```python
from build123d import *

# Parameters (mm, degrees)
F1_DEPTH = 7.5
F3_DEPTH = 7.5
F4_R     = 15
F5_R     = 25
F7_DEPTH = 2


with BuildPart() as f1:
    # F0 (on Front) → F1 (new body, symmetric)
    with BuildSketch(Plane.XZ):
        with BuildLine():
            Line((15.571662, 31.4), (-31.4, 31.4))
            Line((-31.4, 31.4), (-31.4, -31.016811))
            ThreePointArc((-31.4, -31.016811), (-31.146187, -31.209444), (-30.890811, -31.4))
            Line((-30.890811, -31.4), (15.571662, -31.4))
            ThreePointArc((15.571662, -31.4), (31.4, 0), (15.571662, 31.4))
        make_face()
        with BuildLine():
            Line((-21.4, -21.4), (-21.4, 21.4))
            Line((-21.4, 21.4), (12, 21.4))
            ThreePointArc((12, 21.4), (21.4, 0), (12, -21.4))
            Line((12, -21.4), (-21.4, -21.4))
        make_face(mode=Mode.SUBTRACT)
        with BuildLine():
            ThreePointArc((-30.890811, -31.4), (-31.146187, -31.209444), (-31.4, -31.016811))
            Line((-31.4, -31.016811), (-31.4, -31.4))
            Line((-31.4, -31.4), (-30.890811, -31.4))
        make_face()
    extrude(amount=F1_DEPTH, both=True)

    # F2 (on Front) → F3 (join, symmetric)
    with BuildSketch(Plane.XZ):
        with BuildLine():
            ThreePointArc((-71, 31.4), (-93.271008, 0), (-71, -31.4))
            Line((-71, -31.4), (-31.4, -31.4))
            Line((-31.4, -31.4), (-31.4, 6))
            Line((-31.4, 6), (-60, 6))
            Line((-60, 6), (-60, -4))
            Line((-60, -4), (-41.4, -4))
            Line((-41.4, -4), (-41.4, -21.4))
            Line((-41.4, -21.4), (-71, -21.4))
            ThreePointArc((-71, -21.4), (-83.271008, 0), (-71, 21.4))
            Line((-71, 21.4), (-31.4, 21.4))
            Line((-31.4, 21.4), (-31.4, 31.4))
            Line((-31.4, 31.4), (-71, 31.4))
        make_face()
    extrude(amount=F3_DEPTH, both=True)

    # F4
    f4_edges = [f1.edges().sort_by_distance(p)[0] for p in [
        (-71, 0, 21.4),
        (-71, 0, -21.4),
        (12, 0, -21.4),
        (12, 0, 21.4),
    ]]
    fillet(f4_edges, radius=F4_R)

    # F5
    f5_edges = [f1.edges().sort_by_distance(p)[0] for p in [
        (-71, 0, 31.4),
        (-71, 0, -31.4),
        (15.571662, 0, -31.4),
        (15.571662, 0, 31.4),
    ]]
    fillet(f5_edges, radius=F5_R)

    # F6 (on Front) → F7 (cut, symmetric)
    with BuildSketch(Plane.XZ):
        with BuildLine():
            Line((-22.9, 35.188502), (-22.9, 0))
            ThreePointArc((-22.9, 0), (0, -22.9), (22.9, 0))
            Line((22.9, 0), (22.9, 35.188502))
            Line((22.9, 35.188502), (-22.9, 35.188502))
        make_face()
    extrude(amount=F7_DEPTH, both=True, mode=Mode.SUBTRACT)


solid = f1.part
```
Model file for the job. Use its own axes, mm. A direction names the side the tool comes from. Coordinates: 2 decimals unless noted, no trailing zeros. Order: outer loops, then holes, each group sorted by start corner. A loop starts at its lowest first (then second) coordinate and runs counter-clockwise, first axis right, second up. Notation, with made-up numbers: M 52.25,75 L 74.25,75 A30 cw 74.25,109 Z; hole C 30.25,-35 d9. An arc over 180 degrees is marked long. Answer as CSV lines item,"result".
(1) Flat gauge pins, fed straight in: pin 1 (1 mm diameter, centred on x = -80.5, z = -5.5, fed in from +Y); pin 2 (5 mm diameter, centred on y = 0.5, z = -11.5, fed in from +X); pin 3 (2 mm diameter, centred on y = -0.5, z = 11, fed in from -X); pin 4 (4.5 mm diameter, centred on y = -3, z = -15, fed in from -X). Where does each tip first touch, or does it go through?
Geometry says:
pin 1,"passes through"
pin 2,"stops at x = 30.35"
pin 3,"stops at x = -91.73"
pin 4,"stops at x = -90.73"
(2) Band-saw the part on D-D, the plane x = -13.5. List the corners of the cut face in (y, z), then the cut area to 3 significant figures.
Geometry says:
outline,"M -7.5,-31.4 L 7.5,-31.4 L 7.5,-21.4 L -7.5,-21.4 Z; M -7.5,21.4 L -2,21.4 L -2,31.4 L -7.5,31.4 Z; M 2,21.4 L 7.5,21.4 L 7.5,31.4 L 2,31.4 Z"
area,"260 mm2"
(3) Band-saw the part on C-C, the plane z = -6.5. List the corners of the cut face in (x, y).
Geometry says:
outline,"M -92.63,-7.5 L -82.4,-7.5 L -82.4,7.5 L -92.63,7.5 Z; M -41.4,-7.5 L -21.4,-7.5 L -21.4,-2 L -21.96,-2 L -21.96,2 L -21.4,2 L -21.4,7.5 L -41.4,7.5 Z; M 20.66,-7.5 L 30.86,-7.5 L 30.86,7.5 L 20.66,7.5 L 20.66,2 L 21.96,2 L 21.96,-2 L 20.66,-2 Z"
(4) 3-axis set-ups, long thin cutter, end or side, ignore diameter. For faces 5 (the flat face through (0, 2, 22)), 6 (the flat face through (-30, 0, 31.4)), 7 (the cylindrical face through (21.4, -4.8, 0.2)): which of +Z, -Z, +X, -X, +Y, -Y reach the whole face in a straight line?
Geometry says:
face 5,"+Z"
face 6,"+Z, +X, -X, +Y, -Y"
face 7,"+Y, -Y"
(5) Band-saw the part on A-A, the plane y = -0.25. List the corners of the cut face in (x, z), then the cut area to 3 significant figures.
Geometry says:
outline,"M -81.08,-25.74 A25 ccw -65.24,-31.4 L 4.86,-31.4 A25 ccw 27.12,-17.78 A39.06 ccw 27.12,17.78 A25 ccw 22.9,23.71 L 22.9,0 A22.9 cw 16.39,-15.99 A15 cw 11,-20.09 A22.9 cw -8.15,-21.4 L -21.4,-21.4 L -21.4,-8.15 A22.9 cw -22.9,0 L -22.9,31.4 L -65.24,31.4 A25 ccw -81.08,25.74 A33.27 ccw Z; hole M -77.25,-16.2 A15 ccw -65.89,-21.4 L -41.4,-21.4 L -41.4,-4 L -60,-4 L -60,6 L -31.4,6 L -31.4,21.4 L -65.89,21.4 A15 ccw -77.25,16.2 A24.8 ccw Z"
area,"3,220 mm2"
(6) Pull direction X, two halves, no side cores. Call faces 1 (the flat face through (-8, -5, 21.4)), 2 (the cylindrical face through (18.07, 3.438, 27.624)), 3 (the flat face through (1, -2, -22)), 4 (the cylindrical face through (-93.27, -0.11, 0.41)): +X half, -X half, draft (parallel to the pull), parting line (faces both ways), or undercut.
Geometry says:
face 1,"undercut"
face 2,"+X half"
face 3,"undercut"
face 4,"-X half"
(7) Band-saw the part on B-B, the plane x = -37.5. List the corners of the cut face in (y, z).
Geometry says:
outline,"M -7.5,-31.4 L 7.5,-31.4 L 7.5,6 L -7.5,6 Z; M -7.5,21.4 L 7.5,21.4 L 7.5,31.4 L -7.5,31.4 Z"
(8) Wall check: line 1 along Z through (x, y) = (-46.5, 4.25); line 2 along Z through (x, y) = (-13, -4.5); line 3 along Y through (x, z) = (21, -6). Give the ranges that are in metal, low to high.
Geometry says:
line 1,"z = -31.4 to -21.4, -4 to 6, 21.4 to 31.4"
line 2,"z = -31.4 to -21.4, 21.4 to 31.4"
line 3,"y = -7.5 to -2, 2 to 7.5"
